```python
from build123d import *

# Parameters (mm, degrees)
IZIM1_W                     = 72.756230931
IZIM1_H                     = 118.946953667
Y_KSEKLIK_EKSTR_ZYON1_DEPTH = 3
KES_EKSTR_ZYON3_DEPTH       = 4
CUT_EXTRUDE1_DEPTH          = 4


with BuildPart() as part:
    # Çizim1 → Yükseklik-Ekstrüzyon1 (new body)
    with BuildSketch(Plane.XY):
        with Locations((-5.442235915, -33.122673723)):
            Rectangle(IZIM1_W, IZIM1_H)
    extrude(amount=Y_KSEKLIK_EKSTR_ZYON1_DEPTH)

    # Çizim4 → Kes-Ekstrüzyon3 (cut, through all)
    with BuildSketch(Plane(origin=(0, 0, 0), x_dir=(-1, 0, 0), z_dir=(0, 0, -1))):
        with BuildLine():
            Line((20.655005016, -68.253457169), (20.449524021, -67.970805458))
            ThreePointArc((20.449524021, -67.970805458), (20.301021516, -68.004254914), (20.154516787, -68.045585584))
            Line((20.154516787, -68.045585584), (20.108492616, -68.391990267))
            Line((20.108492616, -68.391990267), (20.11956599, -68.588571002))
            ThreePointArc((20.11956599, -68.588571002), (20.074637279, -68.607301226), (20.030106153, -68.62695801))
            Line((20.030106153, -68.62695801), (19.895263796, -68.483486258))
            Line((19.895263796, -68.483486258), (19.612495575, -68.278165626))
            ThreePointArc((19.612495575, -68.278165626), (19.48159775, -68.355867746), (19.355035352, -68.440448001))
            Line((19.355035352, -68.440448001), (19.418308698, -68.784120683))
            Line((19.418308698, -68.784120683), (19.489586891, -68.967658211))
            ThreePointArc((19.489586891, -68.967658211), (19.452645105, -68.999355448), (19.416367768, -69.031811035))
            Line((19.416367768, -69.031811035), (19.243789855, -68.93702987))
            Line((19.243789855, -68.93702987), (18.911413732, -68.829138531))
            ThreePointArc((18.911413732, -68.829138531), (18.810933778, -68.943487291), (18.716702521, -69.063037825))
            Line((18.716702521, -69.063037825), (18.883079748, -69.37033743))
            Line((18.883079748, -69.37033743), (19.007585553, -69.522865819))
            ThreePointArc((19.007585553, -69.522865819), (18.982246812, -69.564427322), (18.957774342, -69.606504734))
            Line((18.957774342, -69.606504734), (18.764354003, -69.569691997))
            Line((18.764354003, -69.569691997), (18.414905268, -69.569791106))
            ThreePointArc((18.414905268, -69.569791106), (18.354678863, -69.709593253), (18.302002759, -69.852411628))
            Line((18.302002759, -69.852411628), (18.555197705, -70.093257528))
            Line((18.555197705, -70.093257528), (18.720743626, -70.199846237))
            ThreePointArc((18.720743626, -70.199846237), (18.709488262, -70.247203677), (18.699216195, -70.294784083))
            Line((18.699216195, -70.294784083), (18.503886761, -70.319543262))
            Line((18.503886761, -70.319543262), (18.17157189, -70.427623118))
            ThreePointArc((18.17157189, -70.427623118), (18.157494415, -70.579193843), (18.151529767, -70.7313))
            Line((18.151529767, -70.7313), (18.466757947, -70.882116522))
            Line((18.466757947, -70.882116522), (18.657139197, -70.932331906))
            ThreePointArc((18.657139197, -70.932331906), (18.661068963, -70.980849606), (18.666002801, -71.029275504))
            Line((18.666002801, -71.029275504), (18.487884476, -71.113182997))
            Line((18.487884476, -71.113182997), (18.205232766, -71.318663992))
            ThreePointArc((18.205232766, -71.318663992), (18.238682221, -71.467166497), (18.280012892, -71.613671226))
            Line((18.280012892, -71.613671226), (18.626417574, -71.659695397))
            Line((18.626417574, -71.659695397), (18.822998309, -71.648622023))
            ThreePointArc((18.822998309, -71.648622023), (18.841728533, -71.693550734), (18.861385317, -71.73808186))
            Line((18.861385317, -71.73808186), (18.717913565, -71.872924217))
            Line((18.717913565, -71.872924217), (18.512592933, -72.155692438))
            ThreePointArc((18.512592933, -72.155692438), (18.590295054, -72.286590263), (18.674875308, -72.413152661))
            Line((18.674875308, -72.413152661), (19.01854799, -72.349879315))
            Line((19.01854799, -72.349879315), (19.202085518, -72.278601122))
            ThreePointArc((19.202085518, -72.278601122), (19.233782755, -72.315542908), (19.266238342, -72.351820245))
            Line((19.266238342, -72.351820245), (19.171457178, -72.524398158))
            Line((19.171457178, -72.524398158), (19.063565838, -72.856774281))
            ThreePointArc((19.063565838, -72.856774281), (19.177914598, -72.957254235), (19.297465133, -73.051485492))
            Line((19.297465133, -73.051485492), (19.604764737, -72.885108265))
            Line((19.604764737, -72.885108265), (19.757293126, -72.76060246))
            ThreePointArc((19.757293126, -72.76060246), (19.79885463, -72.785941201), (19.840932041, -72.810413671))
            Line((19.840932041, -72.810413671), (19.804119305, -73.00383401))
            Line((19.804119305, -73.00383401), (19.804218414, -73.353282745))
            ThreePointArc((19.804218414, -73.353282745), (19.944020561, -73.41350915), (20.086838935, -73.466185254))
            Line((20.086838935, -73.466185254), (20.327684835, -73.212990308))
            Line((20.327684835, -73.212990308), (20.434273545, -73.047444387))
            ThreePointArc((20.434273545, -73.047444387), (20.481630985, -73.058699751), (20.52921139, -73.068971818))
            Line((20.52921139, -73.068971818), (20.553970569, -73.264301252))
            Line((20.553970569, -73.264301252), (20.662050425, -73.596616123))
            ThreePointArc((20.662050425, -73.596616123), (20.813621151, -73.610693598), (20.965727308, -73.616658246))
            Line((20.965727308, -73.616658246), (21.116543829, -73.301430066))
            Line((21.116543829, -73.301430066), (21.166759213, -73.111048816))
            ThreePointArc((21.166759213, -73.111048816), (21.215276914, -73.10711905), (21.263702812, -73.102185212))
            Line((21.263702812, -73.102185212), (21.347610305, -73.280303537))
            Line((21.347610305, -73.280303537), (21.553091299, -73.562955247))
            ThreePointArc((21.553091299, -73.562955247), (21.701593804, -73.529505792), (21.848098533, -73.488175121))
            Line((21.848098533, -73.488175121), (21.894122704, -73.141770439))
            Line((21.894122704, -73.141770439), (21.88304933, -72.945189704))
            ThreePointArc((21.88304933, -72.945189704), (21.927978041, -72.92645948), (21.972509167, -72.906802696))
            Line((21.972509167, -72.906802696), (22.107351525, -73.050274448))
            Line((22.107351525, -73.050274448), (22.390119745, -73.25559508))
            ThreePointArc((22.390119745, -73.25559508), (22.52101757, -73.177892959), (22.647579968, -73.093312705))
            Line((22.647579968, -73.093312705), (22.584306622, -72.749640023))
            Line((22.584306622, -72.749640023), (22.51302843, -72.566102495))
            ThreePointArc((22.51302843, -72.566102495), (22.549970215, -72.534405258), (22.586247553, -72.501949671))
            Line((22.586247553, -72.501949671), (22.758825465, -72.596730835))
            Line((22.758825465, -72.596730835), (23.091201588, -72.704622175))
            ThreePointArc((23.091201588, -72.704622175), (23.191681542, -72.590273415), (23.285912799, -72.47072288))
            Line((23.285912799, -72.47072288), (23.119535572, -72.163423276))
            Line((23.119535572, -72.163423276), (22.995029767, -72.010894887))
            ThreePointArc((22.995029767, -72.010894887), (23.020368508, -71.969333383), (23.044840978, -71.927255972))
            Line((23.044840978, -71.927255972), (23.238261317, -71.964068708))
            Line((23.238261317, -71.964068708), (23.587710053, -71.963969599))
            ThreePointArc((23.587710053, -71.963969599), (23.647936457, -71.824167452), (23.700612562, -71.681349078))
            Line((23.700612562, -71.681349078), (23.447417615, -71.440503178))
            Line((23.447417615, -71.440503178), (23.281871694, -71.333914468))
            ThreePointArc((23.281871694, -71.333914468), (23.293127058, -71.286557028), (23.303399125, -71.238976623))
            Line((23.303399125, -71.238976623), (23.49872856, -71.214217444))
            Line((23.49872856, -71.214217444), (23.83104343, -71.106137588))
            ThreePointArc((23.83104343, -71.106137588), (23.845120905, -70.954566862), (23.851085553, -70.802460705))
            Line((23.851085553, -70.802460705), (23.535857373, -70.651644184))
            Line((23.535857373, -70.651644184), (23.345476123, -70.6014288))
            ThreePointArc((23.345476123, -70.6014288), (23.341546357, -70.552911099), (23.336612519, -70.504485201))
            Line((23.336612519, -70.504485201), (23.514730844, -70.420577708))
            Line((23.514730844, -70.420577708), (23.797382555, -70.215096714))
            ThreePointArc((23.797382555, -70.215096714), (23.763933099, -70.066594209), (23.722602429, -69.92008948))
            Line((23.722602429, -69.92008948), (23.376197746, -69.874065309))
            Line((23.376197746, -69.874065309), (23.179617011, -69.885138683))
            ThreePointArc((23.179617011, -69.885138683), (23.160886787, -69.840209972), (23.141230003, -69.795678846))
            Line((23.141230003, -69.795678846), (23.284701755, -69.660836488))
            Line((23.284701755, -69.660836488), (23.490022387, -69.378068268))
            ThreePointArc((23.490022387, -69.378068268), (23.412320267, -69.247170443), (23.327740012, -69.120608045))
            Line((23.327740012, -69.120608045), (22.98406733, -69.183881391))
            Line((22.98406733, -69.183881391), (22.800529802, -69.255159583))
            ThreePointArc((22.800529802, -69.255159583), (22.768832565, -69.218217798), (22.736376978, -69.18194046))
            Line((22.736376978, -69.18194046), (22.831158143, -69.009362548))
            Line((22.831158143, -69.009362548), (22.939049482, -68.676986425))
            ThreePointArc((22.939049482, -68.676986425), (22.824700722, -68.576506471), (22.705150188, -68.482275214))
            Line((22.705150188, -68.482275214), (22.397850583, -68.648652441))
            Line((22.397850583, -68.648652441), (22.245322194, -68.773158246))
            ThreePointArc((22.245322194, -68.773158246), (22.203760691, -68.747819505), (22.161683279, -68.723347035))
            Line((22.161683279, -68.723347035), (22.198496016, -68.529926696))
            Line((22.198496016, -68.529926696), (22.198396907, -68.18047796))
            ThreePointArc((22.198396907, -68.18047796), (22.05859476, -68.120251556), (21.915776385, -68.067575451))
            Line((21.915776385, -68.067575451), (21.674930485, -68.320770398))
            Line((21.674930485, -68.320770398), (21.568341776, -68.486316319))
            ThreePointArc((21.568341776, -68.486316319), (21.520984336, -68.475060955), (21.47340393, -68.464788888))
            Line((21.47340393, -68.464788888), (21.448644751, -68.269459453))
            Line((21.448644751, -68.269459453), (21.340564895, -67.937144583))
            ThreePointArc((21.340564895, -67.937144583), (21.18899417, -67.923067108), (21.036888013, -67.91710246))
            Line((21.036888013, -67.91710246), (20.886071491, -68.23233064))
            Line((20.886071491, -68.23233064), (20.835856107, -68.42271189))
            ThreePointArc((20.835856107, -68.42271189), (20.787338407, -68.426641656), (20.738912509, -68.431575494))
            Line((20.738912509, -68.431575494), (20.655005016, -68.253457169))
        make_face()
    extrude(amount=-KES_EKSTR_ZYON3_DEPTH, mode=Mode.SUBTRACT)

    # Sketch1 → Cut-Extrude1 (cut, through all)
    with BuildSketch(Plane.XY.offset(3)):
        with BuildLine():
            ThreePointArc((3.32869234, -70.766880353), (-3.797399674, -53.562972367), (-21.00130766, -46.436880353))
            ThreePointArc((-21.00130766, -46.436880353), (-23.75130766, -49.186880353), (-21.00130766, -51.936880353))
            ThreePointArc((-21.00130766, -51.936880353), (-7.68648697, -57.452059663), (-2.17130766, -70.766880353))
            ThreePointArc((-2.17130766, -70.766880353), (0.57869234, -73.516880353), (3.32869234, -70.766880353))
        make_face()
    extrude(amount=-CUT_EXTRUDE1_DEPTH, mode=Mode.SUBTRACT)


solid = part.part
```
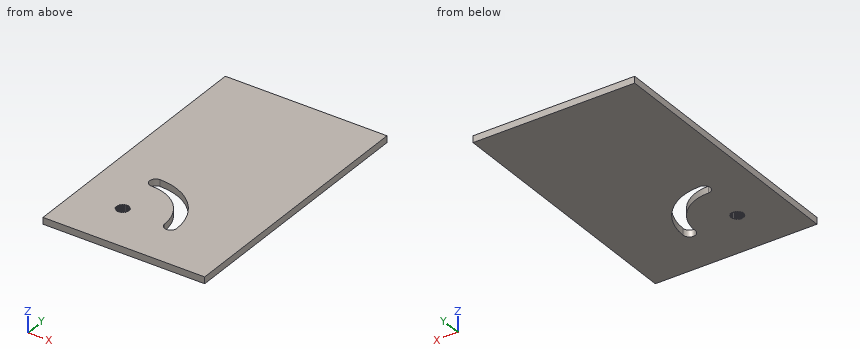
CAD build for the part. Positions are in the model's coordinates, mm. Round coordinates to 2 decimals unless told otherwise and drop trailing zeros. Loops run counter-clockwise (first coordinate to the right, second up) from the corner with the lowest first, then second, coordinate; pieces in that order, holes last. Notation, with made-up numbers: M 79.25,-6 L 121.25,-6 A10 ccw 121.25,-2 Z; hole C 23,64 d2. An arc over 180 degrees is marked long. Use a Markdown table: item, result. Add a question column.
(1) Drill centre lines: line 1 (Y direction, x = -21, z = 2.45); line 2 (X direction, y = -56, z = 1.6); line 3 (Y direction, x = -9.5, z = 0.6). Where is each one in solid material? Low to high.
(2) Cut at A-A (x = -4.5). Give the cut face in (y, z), and give its area (3 significant figures).
(3) Cut at B-B (z = 1.1). State how many separate pieces and enclosed holes the cut face has, and give its area (3 significant figures).
Geometry says:
| question | item | result |
|---|---|---|
| 1 | line 1 | y = -92.6 to -73.55, -67.99 to -51.94, -46.44 to 26.35 |
| 1 | line 2 | x = -41.82 to -9.32, -1.67 to 30.94 |
| 1 | line 3 | y = -92.6 to -55.86, -49.33 to 26.35 |
| 2 | outline | M -92.6,0 L -61.7,0 L -61.7,3 L -92.6,3 Z; M -52.89,0 L 26.35,0 L 26.35,3 L -52.89,3 Z |
| 2 | area | 330 mm² |
| 3 | separate pieces | 1 |
| 3 | enclosed holes | 2 |
| 3 | area | 8,420 mm² |
